```python
from build123d import *

# Parameters (mm, degrees)
SKETCH_1_W          = 57
SKETCH_1_H          = 10
EXTRUDE_1_DEPTH     = 32
SKETCH_2_R          = 5
SKETCH_2_W          = 57
SKETCH_2_H          = 10
EXTRUDE_4_DEPTH     = 28
SKETCH_2_8_R        = 5
SKETCH_2_8_W        = 57
SKETCH_2_8_H        = 10
EXTRUDE_5_DEPTH     = 28
SKETCH_7_W          = 44
SKETCH_7_H          = 2
CUT_EXTRUDE_1_DEPTH = 58.983945463
CUT_EXTRUDE_3_DEPTH = 51.932680387
SKETCH_9_W          = 8
SKETCH_9_H          = 24
CUT_EXTRUDE_4_DEPTH = 20


with BuildPart() as part:
    # 草图1 → 凸台-拉伸1 (new body)
    with BuildSketch(Plane.XY.offset(16)):
        with Locations((-0.085624559, 5)):
            Rectangle(SKETCH_1_W, SKETCH_1_H)
    extrude(amount=-EXTRUDE_1_DEPTH)

    # 草图2 → 凸台-拉伸4 (add)
    # profile 1 of 2: a face of its own
    with BuildSketch(Plane.XY.offset(14)):
        with BuildLine():
            Line((-16.5, 10), (16.5, 10))
            Line((16.5, 10), (10.58774912, 30.983214471))
            ThreePointArc((10.58774912, 30.983214471), (0, 39), (-10.58774912, 30.983214471))
            Line((-10.58774912, 30.983214471), (-16.5, 10))
        make_face()
        with Locations((0, 28)):
            Circle(SKETCH_2_R, mode=Mode.SUBTRACT)
    # profile 2 of 2: a face of its own
    with BuildSketch(Plane.XY.offset(14)):
        with Locations((-0.085624559, 5)):
            Rectangle(SKETCH_2_W, SKETCH_2_H)
    extrude(amount=-EXTRUDE_4_DEPTH)

    # 草图2<8> → 凸台-拉伸5 (add)
    # profile 1 of 2: a face of its own
    with BuildSketch(Plane.XY.offset(14)):
        with BuildLine():
            Line((-16.5, 10), (16.5, 10))
            Line((16.5, 10), (10.58774912, 30.983214471))
            ThreePointArc((10.58774912, 30.983214471), (0, 39), (-10.58774912, 30.983214471))
            Line((-10.58774912, 30.983214471), (-16.5, 10))
        make_face()
        with Locations((0, 28)):
            Circle(SKETCH_2_8_R, mode=Mode.SUBTRACT)
    # profile 2 of 2: a face of its own
    with BuildSketch(Plane.XY.offset(14)):
        with Locations((-0.085624559, 5)):
            Rectangle(SKETCH_2_8_W, SKETCH_2_8_H)
    extrude(amount=-EXTRUDE_5_DEPTH)

    # 草图7 → 切除-拉伸1 (cut, through all)
    with BuildSketch(Plane.XY.offset(16)):
        with Locations((0, 1)):
            Rectangle(SKETCH_7_W, SKETCH_7_H)
    extrude(amount=-CUT_EXTRUDE_1_DEPTH, mode=Mode.SUBTRACT)

    # 草图8 → 切除-拉伸3 (cut, symmetric)
    with BuildSketch(Plane(origin=(0, 0, 0), x_dir=(1, 0, 0), z_dir=(0, 1, 0))):
        with BuildLine():
            Line((-160.076364947, -5), (-28.585624559, -5))
            Line((-28.585624559, -5), (-25.585624559, -5))
            ThreePointArc((-25.585624559, -5), (-20.585624559, 0), (-25.585624559, 5))
            Line((-25.585624559, 5), (-28.585624559, 5))
            Line((-28.585624559, 5), (-160.076364947, 5))
            Line((-160.076364947, 5), (-423.057845722, 5))
            Line((-423.057845722, 5), (-423.057845722, -5))
            Line((-423.057845722, -5), (-160.076364947, -5))
        make_face()
    cut_extrude_3 = extrude(amount=CUT_EXTRUDE_3_DEPTH, both=True, mode=Mode.SUBTRACT)

    # 镜向1: 切除-拉伸3 across plane
    add(cut_extrude_3.mirror(Plane(origin=(0, 0, 0), x_dir=(0, 0, 1), z_dir=(1, 0, 0))), mode=Mode.SUBTRACT)

    # 草图9 → 切除-拉伸4 (cut, symmetric)
    with BuildSketch(Plane(origin=(0, 0, 0), x_dir=(0, 0, -1), z_dir=(1, 0, 0))):
        with Locations((0, 27)):
            Rectangle(SKETCH_9_W, SKETCH_9_H)
    extrude(amount=CUT_EXTRUDE_4_DEPTH, both=True, mode=Mode.SUBTRACT)


solid = part.part
```
Geometry check sheet. Reference: the model listing, model coordinates, mm. A direction names the side the tool comes from. Coordinates: 2 decimals unless noted, no trailing zeros. Loops run counter-clockwise (first coordinate to the right, second up) from the corner with the lowest first, then second, coordinate; pieces in that order, holes last.
Item 1: Release check for a two-part mould opening along X. For faces 6 (the face through (0, 39, -9)), 7 (the face through (-25, 0, 10)), 8 (the face through (-22, 1, 10)) record: released by +X, released by -X, zero draft, split by the parting line, or undercut.
Item 2: Sectioned sample at D-D, the plane y = 28. Record the boundary of the cut face in (x, z).
Item 3: Sectioned sample at C-C, the plane z = -9. Record the boundary of the cut face in (x, y), then the cut area to 3 significant figures.
Item 4: Sectioned sample at A-A, the plane x = 0. Record the boundary of the cut face in (y, z).
Item 5: Access from +Z, -Z, +X, -X, +Y, -Y to the whole of each face (thin tool, end or side, straight path). Record for faces 1 (the face through (0, 2, 0)), 2 (the face through (-27, 5, 5)), 3 (the face through (0, 21, -4)), 4 (the face through (27, 5, 5)), 5 (the face through (-1.08, 23.12, -8.93)).
Item 6: Go/stop test with flat-tipped pins: pin 1 Ø2 at (x, z) = (-4.5, 12.5) entering from -Y; pin 2 Ø2 at (x, z) = (16, -0.5) entering from +Y; pin 3 Ø4 at (y, z) = (24, 3.5) entering from +X. Record where each tip stops, or that it passes through.
Item 7: Thickness scan on line 1 (Z direction, x = 4, y = 23); line 2 (Y direction, x = 0, z = 11); line 3 (Z direction, x = 12, y = 11.5). Record the ranges inside material, lowest first.
Item 8: Sectioned sample at B-B, the plane y = 21. Record the boundary of the cut face in (x, z), then the cut area to 3 significant figures.
Check result:
1. face 6: split by the parting line
1. face 7: zero draft
1. face 8: undercut
2. outline: (-11.43, -14) - (-5, -14) - (-5, -4) - (-11.43, -4) - close; (-11.43, 4) - (-5, 4) - (-5, 14) - (-11.43, 14) - close; (5, -14) - (11.43, -14) - (11.43, -4) - (5, -4) - close; (5, 4) - (11.43, 4) - (11.43, 14) - (5, 14) - close
3. outline: (-28.59, 0) - (-22, 0) - (-22, 2) - (22, 2) - (22, 0) - (28.41, 0) - (28.41, 10) - (16.5, 10) - (10.59, 30.98) arc R11 ccw to (-10.59, 30.98) - (-16.5, 10) - (-28.59, 10) - close; hole circle Ø10 at (0, 28)
3. area: 1,100 mm2
4. outline: (2, -16) - (10, -16) - (10, -14) - (23, -14) - (23, -4) - (15, -4) - (15, 4) - (23, 4) - (23, 14) - (10, 14) - (10, 16) - (2, 16) - close; (33, -14) - (39, -14) - (39, -4) - (33, -4) - close; (33, 4) - (39, 4) - (39, 14) - (33, 14) - close
5. face 1: +Z, -Z, -Y
5. face 2: -X, +Y, -Y
5. face 3: +X, -X, +Y
5. face 4: +X, +Y, -Y
5. face 5: +Z, -Z
6. pin 1: stops at y = 2
6. pin 2: stops at y = 15
6. pin 3: stops at x = 13.1
7. line 1: z = -14 to -4, 4 to 14
7. line 2: y = 2 to 23, 33 to 39
7. line 3: z = -14 to 14
8. outline: (-13.4, -14) - (13.4, -14) - (13.4, -4) - (-13.4, -4) - close; (-13.4, 4) - (13.4, 4) - (13.4, 14) - (-13.4, 14) - close
8. area: 536 mm2
